```python
from build123d import *

# Parameters (mm, degrees)
SWEEP_2_PROFILE_R   = 15
SKETCH_2_R          = 40
EXTRUDE_1_DEPTH     = 10
SWEEP_4_PROFILE_R   = 45
SWEEP_6_PROFILE_R   = 10
SWEEP_2_2_PROFILE_R = 12
SKETCH_7_R          = 4.5
CUT_EXTRUDE_1_DEPTH = 10
SWEEP_14_PROFILE_R  = 5.5
SWEEP_16_PROFILE_R  = 5.5
SWEEP_18_PROFILE_R  = 5.5
SWEEP_20_PROFILE_R  = 5.5
SWEEP_24_PROFILE_R  = 7


with BuildPart() as part:
    # Sweep 2: sweep along a curve in space
    with BuildLine() as sweep_2_path:
        Line((0, 0, 0), (105, 0, 0))
        ThreePointArc((105, 0, 0), (136.819805153, 13.180194847, 0), (150, 45, 0))
        Line((150, 45, 0), (150, 82.789579623, 0))
        ThreePointArc((150, 82.789579623, 0), (154.47011502, 114.412356225, 7.822701285), (166.537964612, 136.537964612, 28.941438071))
        Line((166.537964612, 136.537964612, 28.941438071), (230, 200, 140))
    # Sweep 2 profile (on start of the path) → Sweep 2 (sweep)
    with BuildSketch(Plane(origin=(0, 0, 0), x_dir=(0, 0, 1), z_dir=(1, 0, 0))):
        Circle(SWEEP_2_PROFILE_R)
    sweep(path=sweep_2_path.line)

    # 草图2 → 凸台-拉伸1 (add)
    with BuildSketch(Plane(origin=(0, 0, 0), x_dir=(0, 0, -1), z_dir=(1, 0, 0))):
        Circle(SKETCH_2_R)
    extrude(amount=EXTRUDE_1_DEPTH)

    # 扫描4: sweep along a curve in space
    with BuildLine() as sweep_4_path:
        Line((230, 200, 140), (224.666667, 194.666667, 130.666667))
    # 扫描4 profile (on start of the path) → 扫描4 (sweep)
    with BuildSketch(Plane(origin=(230, 200, 140), x_dir=(-0.8682431478491394, 0, 0.4961389283386436), z_dir=(-0.4444444372427982, -0.4444444372427982, -0.7777777860082306))):
        Circle(SWEEP_4_PROFILE_R)
    sweep(path=sweep_4_path.line)

    # 扫描6: sweep along a curve in space
    with BuildLine() as sweep_6_path:
        Line((150, 60, -5), (150, 60, -70))
    # 扫描6 profile (on start of the path) → 扫描6 (sweep)
    with BuildSketch(Plane(origin=(150, 60, -5), x_dir=(-1, 0, 0), z_dir=(0, 0, -1))):
        Circle(SWEEP_6_PROFILE_R)
    sweep(path=sweep_6_path.line)

    # Sweep 2 2: sweep along a curve in space
    with BuildLine() as sweep_2_2_path:
        Line((-5, 0, 0), (105, 0, 0))
        ThreePointArc((105, 0, 0), (136.819805153, 13.180194847, 0), (150, 45, 0))
        Line((150, 45, 0), (150, 82.789575291, 0))
        ThreePointArc((150, 82.789575291, 0), (154.470114667, 114.412354552, 7.822703386), (166.537963061, 136.537963061, 28.941445413))
        Line((166.537963061, 136.537963061, 28.941445413), (232.2222, 202.2222, 143.8889))
    # Sweep 2 2 profile (on start of the path) → Sweep 2 2 (sweep, cut)
    with BuildSketch(Plane(origin=(-5, 0, 0), x_dir=(0, 0, 1), z_dir=(1, 0, 0))):
        Circle(SWEEP_2_2_PROFILE_R)
    sweep(path=sweep_2_2_path.line, mode=Mode.SUBTRACT)

    # 草图7 → 切除-拉伸1 (cut)
    with BuildSketch(Plane(origin=(0, 0, 0), x_dir=(0, 0, -1), z_dir=(1, 0, 0))):
        with Locations((-21.2132, 21.2132)):
            Circle(SKETCH_7_R)
        with Locations((21.2132, 21.2132)):
            Circle(SKETCH_7_R)
        with Locations((21.2132, -21.2132)):
            Circle(SKETCH_7_R)
        with Locations((-21.2132, -21.2132)):
            Circle(SKETCH_7_R)
    extrude(amount=CUT_EXTRUDE_1_DEPTH, mode=Mode.SUBTRACT)

    # 切除-扫描14: sweep along a curve in space
    with BuildLine() as sweep_14_path:
        Line((196.713944, 214.424944, 130.205492), (205.602764, 223.313764, 145.761127))
    # 切除-扫描14 profile (on start of the path) → 切除-扫描14 (sweep, cut)
    with BuildSketch(Plane(origin=(196.713944, 214.424944, 130.205492), x_dir=(0.8682458899522337, 0, -0.4961341296273152), z_dir=(0.4444409876456375, 0.4444409876456375, 0.777781728379589))):
        Circle(SWEEP_14_PROFILE_R)
    sweep(path=sweep_14_path.line, mode=Mode.SUBTRACT)

    # 切除-扫描16: sweep along a curve in space
    with BuildLine() as sweep_16_path:
        Line((238.461944, 214.424944, 106.350492), (247.350764, 223.313764, 121.906127))
    # 切除-扫描16 profile (on start of the path) → 切除-扫描16 (sweep, cut)
    with BuildSketch(Plane(origin=(238.461944, 214.424944, 106.350492), x_dir=(0.8682458899522337, 0, -0.4961341296273152), z_dir=(0.4444409876456375, 0.4444409876456375, 0.777781728379589))):
        Circle(SWEEP_16_PROFILE_R)
    sweep(path=sweep_16_path.line, mode=Mode.SUBTRACT)

    # 切除-扫描18: sweep along a curve in space
    with BuildLine() as sweep_18_path:
        Line((207.315944, 171.352944, 148.760492), (216.204764, 180.241764, 164.316127))
    # 切除-扫描18 profile (on start of the path) → 切除-扫描18 (sweep, cut)
    with BuildSketch(Plane(origin=(207.315944, 171.352944, 148.760492), x_dir=(0.8682458899522337, 0, -0.4961341296273152), z_dir=(0.4444409876456375, 0.4444409876456375, 0.777781728379589))):
        Circle(SWEEP_18_PROFILE_R)
    sweep(path=sweep_18_path.line, mode=Mode.SUBTRACT)

    # 切除-扫描20: sweep along a curve in space
    with BuildLine() as sweep_20_path:
        Line((249.063944, 171.352944, 124.905492), (257.952764, 180.241764, 140.461127))
    # 切除-扫描20 profile (on start of the path) → 切除-扫描20 (sweep, cut)
    with BuildSketch(Plane(origin=(249.063944, 171.352944, 124.905492), x_dir=(0.8682458899522337, 0, -0.4961341296273152), z_dir=(0.4444409876456375, 0.4444409876456375, 0.777781728379589))):
        Circle(SWEEP_20_PROFILE_R)
    sweep(path=sweep_20_path.line, mode=Mode.SUBTRACT)

    # 切除-扫描24: sweep along a curve in space
    with BuildLine() as sweep_24_path:
        Line((150, 60, 10), (150, 60, -70))
    # 切除-扫描24 profile (on start of the path) → 切除-扫描24 (sweep, cut)
    with BuildSketch(Plane(origin=(150, 60, 10), x_dir=(-1, 0, 0), z_dir=(0, 0, -1))):
        Circle(SWEEP_24_PROFILE_R)
    sweep(path=sweep_24_path.line, mode=Mode.SUBTRACT)


solid = part.part
```
Build history of the part. All positions in model axes, mm. A direction names the side the tool comes from. Round coordinates to 2 decimals unless told otherwise and drop trailing zeros.
1) Pin check, flat tips, straight feed: pin 1 (8.5 mm diameter, centred on x = 150, y = 60, fed in from +Z); pin 2 (4 mm diameter, centred on y = 117.5, z = -6.5, fed in from +X); pin 3 (14.5 mm diameter, centred on y = 21.21, z = 21.21, fed in from -X); pin 4 (11.5 mm diameter, centred on y = -21.21, z = -21.21, fed in from +X). Stop position of each tip, or through.
2) Band-saw the part on A-A, the plane z = 29.5. Give the number of separate pieces and of enclosed holes in the cut face, and give its area (3 significant figures).
3) Mould opens along Y. For faces 4 (the cylindrical face through (4.93, 24.255, 24.53)), 5 (the flat face through (0, -8.3, 9.4)), 6 (the cylindrical face through (207.83, 171.99, 78.17)), 7 (the cylindrical face through (58.165, -0.66, -14.985)) say: +Y half, -Y half, draft (parallel to the pull), parting line (faces both ways), or undercut.
4) 3-axis set-ups, long thin cutter, end or side, ignore diameter. For faces 1 (the cylindrical face through (53.24, -0.53, -11.99)), 2 (the flat face through (148, 67, -70)), 3 (the cylindrical face through (153.604, 64.159, 11.446)): which of +Z, -Z, +X, -X, +Y, -Y reach the whole face in a straight line?
5) Drill centre lines: probe 1 along X at (y, z) = (70, 0); probe 2 along X at (y, z) = (151, 57.5); probe 3 along Z at (x, y) = (150, 64). Where is each one in solid material? Low to high.
Ans:
1. pin 1: stops at z = 15
1. pin 2: stops at x = 162.63
1. pin 3: stops at x = 0
1. pin 4: stops at x = 10
2. separate pieces: 2
2. enclosed holes: 1
2. area: 881 mm2
3. face 4: undercut
3. face 5: draft
3. face 6: undercut
3. face 7: parting line
4. face 1: -X
4. face 2: -Z, +X, -X, +Y, -Y
4. face 3: none
5. probe 1: x = 135 to 138, 162 to 165
5. probe 2: x = 165.75 to 169.13, 195.67 to 199.05
5. probe 3: z = 12 to 15
